```python
from build123d import *

# Parameters (mm, degrees)
F0_R     = 6.35
F1_DEPTH = 88.9
F2_W     = 44.45
F2_H     = 88.9
F3_DEPTH = 101.6


with BuildPart() as f1:
    # F0 (on Front) → F1 (new body)
    with BuildSketch(Plane.XZ):
        Polygon((44.45, 88.9), (44.45, 177.8), (-44.45, 177.8), (-44.45, -177.8), (19.05, -177.8), align=None)
        with Locations((0, 114.3)):
            Circle(F0_R, mode=Mode.SUBTRACT)
        with Locations((0, 152.4)):
            Circle(F0_R, mode=Mode.SUBTRACT)
    extrude(amount=F1_DEPTH)

    # F2 (on face) → F3 (cut)
    with BuildSketch(Plane.YZ.offset(44.45)):
        with Locations((-22.225, 133.35)):
            Rectangle(F2_W, F2_H)
    extrude(amount=-F3_DEPTH, mode=Mode.SUBTRACT)


solid = f1.part
```
Geometry check sheet. Reference: the model listing, model coordinates, mm. A direction names the side the tool comes from. Coordinates: 2 decimals unless noted, no trailing zeros. Order: outer loops, then holes, each group sorted by start corner. A loop starts at its lowest first (then second) coordinate and runs counter-clockwise, first axis right, second up. Notation, with made-up numbers: M -10,-22.75 L 46,-22.75 A15 cw 46,-7.75 Z; hole C 68.5,80.5 d6. An arc over 180 degrees is marked long. One line per question, with ' | ' between items. Start each with the question number.
Item 1: Cross-section at D-D on x = -17.5. Enter the section's corners in (y, z).
Item 2: Gauge pin test, flat ends, axial feed: pin 1 (4 mm diameter, centred on x = 33, z = 80, fed in from +Y); pin 2 (12 mm diameter, centred on y = -39, z = -109, fed in from +X); pin 3 (7.5 mm diameter, centred on x = 0, z = 152.4, fed in from +Y); pin 4 (14.5 mm diameter, centred on x = 0, z = 114.3, fed in from +Y). Record the tip position at first contact, or that the pin passes through.
Item 3: Cross-section at B-B on y = -61. Enter the section's corners in (x, z), then the cut area to 3 significant figures.
Item 4: Cross-section at A-A on z = 152.4. Enter the section's corners in (x, y).
Item 5: Cross-section at C-C on x = 0. Enter the section's corners in (y, z), then the cut area to 3 significant figures.
Item 6: Set-up check for faces 4 (the flat face through (1, -44.45, 133)), 5 (the flat face through (-44.45, -44, 2)): record each of +Z, -Z, +X, -X, +Y, -Y from which the full face is reachable in a straight line by a thin tool's end or side.
Item 7: Draft check along X on faces 1 (the cylindrical face through (-1.38, -66.36, 108.1)), 2 (the flat face through (-1, -88.9, 2)), 3 (the flat face through (31.57, -43.83, -46.32)). Enter one of: pulls with the +X half, pulls with the -X half, needs draft (parallel to the pull), parting line crosses it, or undercut.
Item 8: Material ranges on L1, parallel to Z at x = 0, y = -55; L2, parallel to X at y = -77, z = 152; L3, parallel to Z at x = 6, y = -40, recorded low to high. Write a range as [from, to].
Findings:
1) outline: M -88.9,-177.8 L 0,-177.8 L 0,88.9 L -44.45,88.9 L -44.45,177.8 L -88.9,177.8 Z
2) pin 1: stops at y = 0 | pin 2: stops at x = 26.17 | pin 3: passes through | pin 4: stops at y = -44.45
3) outline: M -44.45,-177.8 L 19.05,-177.8 L 44.45,88.9 L 44.45,177.8 L -44.45,177.8 Z; hole C 0,114.3 d12.7; hole C 0,152.4 d12.7 | area: 28,000 mm²
4) outline: M -44.45,-88.9 L -6.35,-88.9 L -6.35,-44.45 L -44.45,-44.45 Z; M 6.35,-88.9 L 44.45,-88.9 L 44.45,-44.45 L 6.35,-44.45 Z
5) outline: M -88.9,-177.8 L 0,-177.8 L 0,88.9 L -44.45,88.9 L -44.45,107.95 L -88.9,107.95 Z; M -88.9,120.65 L -44.45,120.65 L -44.45,146.05 L -88.9,146.05 Z; M -88.9,158.75 L -44.45,158.75 L -44.45,177.8 L -88.9,177.8 Z | area: 26,500 mm²
6) face 4: +Z, +X, -X, +Y | face 5: +Z, -Z, -X, +Y, -Y
7) face 1: undercut | face 2: needs draft | face 3: pulls with the +X half
8) L1: z = [-177.8, 107.95], [120.65, 146.05], [158.75, 177.8] | L2: x = [-44.45, -6.34], [6.34, 44.45] | L3: z = [-177.8, 88.9]
